Read the model definition and answer for the solid it produces. Units are mm, in the model's axes. A direction names the side the tool comes from. Coordinates: 2 decimals unless noted, no trailing zeros. Loops run counter-clockwise (first coordinate to the right, second up) from the corner with the lowest first, then second, coordinate; pieces in that order, holes last. Notation, with made-up numbers: (74.5, 32) - (116.5, 32) arc R17 ccw to (116.5, 39) - close; hole circle Ø2 at (-36, 74.5). An arc over 180 degrees is marked (long way). Use one line per item in the form item = value.
from build123d import *

# Parameters (mm, degrees)
SKETCH1_W            = 81.28
SKETCH1_H            = 81.28
SKETCH1_W_2          = 76.2
SKETCH1_H_2          = 76.2
BOSS_EXTRUDE1_DEPTH  = 177.8
SKETCH2_W            = 2.54
SKETCH2_H            = 38.1
BOSS_EXTRUDE2_DEPTH  = 25.4
SKETCH3_W            = 2.54
SKETCH3_H            = 25.4
CUT_EXTRUDE1_DEPTH   = 212.720846399
BOSS_EXTRUDE3_DEPTH  = 12.7
BOSS_EXTRUDE4_DEPTH  = 12.7
SKETCH14_W           = 5.08
SKETCH14_H           = 25.4
BOSS_EXTRUDE6_DEPTH  = 76.2
CUT_EXTRUDE2_REACH   = 243.407
SKETCH16_W           = 23.13
SKETCH16_H           = 20.32
SKETCH22_R           = 2
CUT_EXTRUDE6_DEPTH   = 252.036309724
SKETCH28_W           = 35.399999812
SKETCH28_H           = 50.8
BOSS_EXTRUDE7_DEPTH  = 38.1
CUT_EXTRUDE8_REACH   = 246.574
SKETCH32_W           = 33.02
SKETCH32_H           = 30.319999812
CUT_EXTRUDE9_DEPTH   = 25.4
CUT_EXTRUDE13_REACH  = 245.27
SKETCH34_R           = 9.890000016
BOSS_EXTRUDE9_DEPTH  = 2.54
SKETCH38_W           = 2.54
SKETCH38_H           = 25.4
CUT_EXTRUDE15_DEPTH  = 63.5
CUT_EXTRUDE17_REACH  = 224.71
SKETCH40_R           = 2.999995
SKETCH41_R           = 3.77
SKETCH41_R_2         = 2.5
BOSS_EXTRUDE10_DEPTH = 5
BOSS_EXTRUDE11_START = 5
SKETCH42_R           = 3.77
SKETCH42_R_2         = 2.5
BOSS_EXTRUDE11_DEPTH = 5
SKETCH43_W           = 76.2
SKETCH43_H           = 76.2
CUT_EXTRUDE20_DEPTH  = 25.4
SKETCH44_W           = 174.6
SKETCH44_H           = 70
SKETCH44_R           = 1.5
BOSS_EXTRUDE12_DEPTH = 2.54
FILLET1_R            = 5.08
FILLET2_R            = 12.7
FILLET3_R            = 2.54
FILLET7_R            = 12.7
FILLET9_R            = 12.7
BOSS_EXTRUDE20_DEPTH = 88.9
CUT_EXTRUDE21_REACH  = 275.109
SKETCH54_R           = 2.5
SKETCH55_W           = 30.48
SKETCH55_H           = 33.02
BOSS_EXTRUDE21_DEPTH = 2.54
FILLET12_R           = 2.54
FILLET13_R           = 2.54


with BuildPart() as part:
    # Sketch1 → Boss-Extrude1 (new body)
    with BuildSketch(Plane(origin=(0, 0, 0), x_dir=(1, 0, 0), z_dir=(0, 1, 0))):
        with Locations((40.64, 40.64)):
            Rectangle(SKETCH1_W, SKETCH1_H)
        with Locations((40.64, 40.64)):
            Rectangle(SKETCH1_W_2, SKETCH1_H_2, mode=Mode.SUBTRACT)
    extrude(amount=BOSS_EXTRUDE1_DEPTH)

    # Sketch2 → Boss-Extrude2 (add)
    with BuildSketch(Plane(origin=(0, 0, 0), x_dir=(0, 0, -1), z_dir=(1, 0, 0))):
        with Locations((64.77, 19.05)):
            Rectangle(SKETCH2_W, SKETCH2_H)
    extrude(amount=-BOSS_EXTRUDE2_DEPTH)

    # Sketch3 → Cut-Extrude1 (cut, through all)
    with BuildSketch(Plane.XY):
        with Locations((80.01, 12.7)):
            Rectangle(SKETCH3_W, SKETCH3_H)
    extrude(amount=-CUT_EXTRUDE1_DEPTH, mode=Mode.SUBTRACT)

    # Sketch7 → Boss-Extrude3 (add)
    with BuildSketch(Plane.XY):
        Polygon((81.28, 25.4), (106.68, 50.8), (81.28, 50.8), align=None)
    extrude(amount=-BOSS_EXTRUDE3_DEPTH)

    # Sketch10 → Boss-Extrude4 (add)
    with BuildSketch(Plane(origin=(0, 0, -81.28), x_dir=(-1, 0, 0), z_dir=(0, 0, -1))):
        Polygon((-81.28, 25.4), (-81.28, 50.8), (-106.68, 50.8), align=None)
    extrude(amount=-BOSS_EXTRUDE4_DEPTH)

    # Sketch14 → Boss-Extrude6 (add)
    with BuildSketch(Plane(origin=(81.28, 0, 0), x_dir=(0, 0, -1), z_dir=(1, 0, 0))):
        with Locations((40.64, 38.1)):
            Rectangle(SKETCH14_W, SKETCH14_H)
    extrude(amount=BOSS_EXTRUDE6_DEPTH)

    # Sketch16 → Cut-Extrude2 (cut, up to next)
    with BuildSketch(Plane.XY.offset(-38.1), mode=Mode.PRIVATE) as cut_extrude2_sk1:
        with Locations((129.405, 40.64)):
            Rectangle(SKETCH16_W, SKETCH16_H)
    cut_extrude2_tool1 = extrude(cut_extrude2_sk1.sketch, amount=-CUT_EXTRUDE2_REACH, mode=Mode.PRIVATE) & part.part
    add(cut_extrude2_tool1.solids().sort_by_distance((129.405, 40.64, -38.1))[0], mode=Mode.SUBTRACT)

    # Sketch22 → Cut-Extrude6 (cut, through all)
    with BuildSketch(Plane.XY):
        with Locations((93.98, 45.72)):
            Circle(SKETCH22_R)
    extrude(amount=-CUT_EXTRUDE6_DEPTH, mode=Mode.SUBTRACT)

    # Sketch28 → Boss-Extrude7 (add)
    with BuildSketch(Plane(origin=(81.28, 0, 0), x_dir=(0, 0, -1), z_dir=(1, 0, 0))):
        with Locations((40.64, 152.4)):
            Rectangle(SKETCH28_W, SKETCH28_H)
    extrude(amount=BOSS_EXTRUDE7_DEPTH)

    # Sketch30 → Cut-Extrude8 (cut, up to next)
    with BuildSketch(Plane.XY.offset(-22.940000094), mode=Mode.PRIVATE) as cut_extrude8_sk1:
        Polygon((81.28, 127), (119.38, 127), (119.38, 152.4), align=None)
    cut_extrude8_tool1 = extrude(cut_extrude8_sk1.sketch, amount=-CUT_EXTRUDE8_REACH, mode=Mode.PRIVATE) & part.part
    add(cut_extrude8_tool1.solids().sort_by_distance((106.68, 135.466667, -22.94))[0], mode=Mode.SUBTRACT)

    # Sketch32 → Cut-Extrude9 (cut)
    with BuildSketch(Plane(origin=(0, 177.8, 0), x_dir=(1, 0, 0), z_dir=(0, 1, 0))):
        with Locations((100.33, 40.64)):
            Rectangle(SKETCH32_W, SKETCH32_H)
    extrude(amount=-CUT_EXTRUDE9_DEPTH, mode=Mode.SUBTRACT)

    # Cut-Extrude13: up to this face of the body (flat: up to its plane)
    cut_extrude13_end = Plane(part.part.faces().sort_by_distance((78.74, 101.6, -40.64))[0])
    # Sketch34 → Cut-Extrude13 (cut, up to the picked face)
    with BuildSketch(Plane(origin=(119.38, 0, 0), x_dir=(0, 0, -1), z_dir=(1, 0, 0)), mode=Mode.PRIVATE) as cut_extrude13_sk1:
        with Locations(Location((40.593000094, 165.1, 0), (0, 0, 180))):
            Circle(SKETCH34_R)
    cut_extrude13_tool1 = split(extrude(cut_extrude13_sk1.sketch, amount=-CUT_EXTRUDE13_REACH, mode=Mode.PRIVATE), bisect_by=cut_extrude13_end, keep=Keep.BOTH, mode=Mode.PRIVATE)
    add(cut_extrude13_tool1.solids().sort_by(Axis((119.38, 165.1, -40.593), (-1, 0, 0)))[0], mode=Mode.SUBTRACT)

    # Sketch37 → Boss-Extrude9 (add)
    with BuildSketch(Plane.XY.offset(-63.5)):
        Polygon((-25.4, 38.1), (0, 38.1), (0, 52.764696837), align=None)
    extrude(amount=-BOSS_EXTRUDE9_DEPTH)

    # Sketch38 → Cut-Extrude15 (cut)
    with BuildSketch(Plane.XY):
        with Locations((1.27, 12.7)):
            Rectangle(SKETCH38_W, SKETCH38_H)
    extrude(amount=-CUT_EXTRUDE15_DEPTH, mode=Mode.SUBTRACT)

    # Cut-Extrude17: up to this face of the body (flat: up to its plane)
    cut_extrude17_end = Plane(part.part.faces().sort_by_distance((0, 99.23335202, -41.514066738))[0])
    # Sketch40 → Cut-Extrude17 (cut, up to the picked face)
    with BuildSketch(Plane(origin=(81.28, 0, 0), x_dir=(0, 0, -1), z_dir=(1, 0, 0)), mode=Mode.PRIVATE) as cut_extrude17_sk1:
        with Locations((19.05, 101.6)):
            Circle(SKETCH40_R)
    cut_extrude17_tool1 = split(extrude(cut_extrude17_sk1.sketch, amount=-CUT_EXTRUDE17_REACH, mode=Mode.PRIVATE), bisect_by=cut_extrude17_end, keep=Keep.BOTH, mode=Mode.PRIVATE)
    # Sketch40 → Cut-Extrude17 (cut, up to the picked face)
    with BuildSketch(Plane(origin=(81.28, 0, 0), x_dir=(0, 0, -1), z_dir=(1, 0, 0)), mode=Mode.PRIVATE) as cut_extrude17_sk2:
        with Locations((62.23, 101.6)):
            Circle(SKETCH40_R)
    cut_extrude17_tool2 = split(extrude(cut_extrude17_sk2.sketch, amount=-CUT_EXTRUDE17_REACH, mode=Mode.PRIVATE), bisect_by=cut_extrude17_end, keep=Keep.BOTH, mode=Mode.PRIVATE)
    add(cut_extrude17_tool1.solids().sort_by(Axis((81.28, 101.6, -19.05), (-1, 0, 0)))[0], mode=Mode.SUBTRACT)
    add(cut_extrude17_tool2.solids().sort_by(Axis((81.28, 101.6, -62.23), (-1, 0, 0)))[0], mode=Mode.SUBTRACT)

    # Sketch41 → Boss-Extrude10 (add)
    # profile 1 of 2: a face of its own
    with BuildSketch(Plane(origin=(81.28, 0, 0), x_dir=(0, 0, -1), z_dir=(1, 0, 0))):
        with Locations(Location((19.05, 101.6, 0), (0, 0, 180))):
            Circle(SKETCH41_R)
        with Locations((19.05, 101.6)):
            Circle(SKETCH41_R_2, mode=Mode.SUBTRACT)
    # profile 2 of 2: a face of its own
    with BuildSketch(Plane(origin=(81.28, 0, 0), x_dir=(0, 0, -1), z_dir=(1, 0, 0))):
        with Locations(Location((62.23, 101.6, 0), (0, 0, 180))):
            Circle(SKETCH41_R)
        with Locations((62.23, 101.6)):
            Circle(SKETCH41_R_2, mode=Mode.SUBTRACT)
    extrude(amount=BOSS_EXTRUDE10_DEPTH)

    # Sketch42 → Boss-Extrude11 (add)
    # profile 1 of 2: a face of its own
    with BuildSketch(Plane.ZY.offset(BOSS_EXTRUDE11_START)):
        with Locations((-62.23, 101.6)):
            Circle(SKETCH42_R)
        with Locations(Location((-62.23, 101.6, 0), (0, 0, 180))):
            Circle(SKETCH42_R_2, mode=Mode.SUBTRACT)
    # profile 2 of 2: a face of its own
    with BuildSketch(Plane.ZY.offset(BOSS_EXTRUDE11_START)):
        with Locations((-19.05, 101.6)):
            Circle(SKETCH42_R)
        with Locations(Location((-19.05, 101.6, 0), (0, 0, 180))):
            Circle(SKETCH42_R_2, mode=Mode.SUBTRACT)
    extrude(amount=-BOSS_EXTRUDE11_DEPTH)

    # Sketch43 → Cut-Extrude20 (cut)
    with BuildSketch(Plane(origin=(0, 177.8, 0), x_dir=(1, 0, 0), z_dir=(0, 1, 0))):
        Polygon((83.82, 58.339999906), (83.82, 22.940000094), (81.28, 22.940000094), (81.28, 0), (0, 0), (0, 81.28), (81.28, 81.28), (81.28, 58.339999906), align=None)
        with Locations((40.64, 40.64)):
            Rectangle(SKETCH43_W, SKETCH43_H, mode=Mode.SUBTRACT)
    extrude(amount=-CUT_EXTRUDE20_DEPTH, mode=Mode.SUBTRACT)

    # Sketch44 → Boss-Extrude12 (add)
    with BuildSketch(Plane.XY):
        with Locations((87.3, 85.8)):
            Rectangle(SKETCH44_W, SKETCH44_H)
        with Locations((140.97, 115.8)):
            Circle(SKETCH44_R, mode=Mode.SUBTRACT)
        with Locations((140.97, 55.8)):
            Circle(SKETCH44_R, mode=Mode.SUBTRACT)
    extrude(amount=-BOSS_EXTRUDE12_DEPTH)

    # Fillet1
    fillet1_edges = [part.edges().sort_by_distance(p)[0] for p in [
        (106.68, 50.8, -7.62),
        (106.68, 50.8, -74.93),
    ]]
    fillet(fillet1_edges, radius=FILLET1_R)

    # Fillet2
    fillet2_edges = [part.edges().sort_by_distance(p)[0] for p in [
        (174.6, 120.8, -1.27),
        (174.6, 50.8, -1.27),
    ]]
    fillet(fillet2_edges, radius=FILLET2_R)

    # Fillet3
    fillet3_edges = [part.edges().sort_by_distance(p)[0] for p in [
        (157.48, 50.8, -40.64),
        (157.48, 25.4, -40.64),
    ]]
    fillet(fillet3_edges, radius=FILLET3_R)

    # Fillet7
    fillet7_edges = [part.edges().sort_by_distance(p)[0] for p in [
        (-25.4, 38.1, -64.77),
    ]]
    fillet(fillet7_edges, radius=FILLET7_R)

    # Fillet9
    fillet9_edges = [part.edges().sort_by_distance(p)[0] for p in [
        (83.82, 177.8, -24.210000094),
        (83.82, 177.8, -57.069999906),
    ]]
    fillet(fillet9_edges, radius=FILLET9_R)

    # Sketch53 → Boss-Extrude20 (add)
    with BuildSketch(Plane(origin=(0, 0, 0), x_dir=(-1, 0, 0), z_dir=(0, -1, 0))):
        Polygon((-35.659105782, 81.28), (-35.659105782, 78.74), (-45.72, 78.74), (-45.72, 111.76), (-15.24, 111.76), (-15.24, 106.68), (-40.64, 106.68), (-40.64, 81.28), align=None)
    extrude(amount=-BOSS_EXTRUDE20_DEPTH)

    # Sketch54 → Cut-Extrude21 (cut, up to next)
    with BuildSketch(Plane(origin=(0, 0, -111.76), x_dir=(-1, 0, 0), z_dir=(0, 0, -1)), mode=Mode.PRIVATE) as cut_extrude21_sk1:
        with Locations((-30.48, 76.2)):
            Circle(SKETCH54_R)
    cut_extrude21_tool1 = extrude(cut_extrude21_sk1.sketch, amount=-CUT_EXTRUDE21_REACH, mode=Mode.PRIVATE) & part.part
    # Sketch54 → Cut-Extrude21 (cut, up to next)
    with BuildSketch(Plane(origin=(0, 0, -111.76), x_dir=(-1, 0, 0), z_dir=(0, 0, -1)), mode=Mode.PRIVATE) as cut_extrude21_sk2:
        with Locations((-30.48, 44.45)):
            Circle(SKETCH54_R)
    cut_extrude21_tool2 = extrude(cut_extrude21_sk2.sketch, amount=-CUT_EXTRUDE21_REACH, mode=Mode.PRIVATE) & part.part
    # Sketch54 → Cut-Extrude21 (cut, up to next)
    with BuildSketch(Plane(origin=(0, 0, -111.76), x_dir=(-1, 0, 0), z_dir=(0, 0, -1)), mode=Mode.PRIVATE) as cut_extrude21_sk3:
        with Locations((-30.48, 12.7)):
            Circle(SKETCH54_R)
    cut_extrude21_tool3 = extrude(cut_extrude21_sk3.sketch, amount=-CUT_EXTRUDE21_REACH, mode=Mode.PRIVATE) & part.part
    add(cut_extrude21_tool1.solids().sort_by_distance((30.48, 76.2, -111.76))[0], mode=Mode.SUBTRACT)
    add(cut_extrude21_tool2.solids().sort_by_distance((30.48, 44.45, -111.76))[0], mode=Mode.SUBTRACT)
    add(cut_extrude21_tool3.solids().sort_by_distance((30.48, 12.7, -111.76))[0], mode=Mode.SUBTRACT)

    # Sketch55 → Boss-Extrude21 (add)
    with BuildSketch(Plane(origin=(0, 0, 0), x_dir=(-1, 0, 0), z_dir=(0, -1, 0))):
        with Locations((-30.48, 95.25)):
            Rectangle(SKETCH55_W, SKETCH55_H)
    extrude(amount=-BOSS_EXTRUDE21_DEPTH)

    # Fillet12
    fillet12_edges = [part.edges().sort_by_distance(p)[0] for p in [
        (81.28, 136.6, 0),
        (81.28, 101.6, -81.28),
        (0, 76.2, -81.28),
        (0, 88.9, 0),
    ]]
    fillet(fillet12_edges, radius=FILLET12_R)

    # Fillet13
    fillet13_edges = [part.edges().sort_by_distance(p)[0] for p in [
        (15.24, 45.72, -106.68),
        (15.24, 44.45, -111.76),
    ]]
    fillet(fillet13_edges, radius=FILLET13_R - 0.0001)  # a hair under: the kernel refuses the full size


solid = part.part
Item 1: For a pull along Y with two mould halves and no side action, classify faces 1 (the cylindrical face through (118.128, 174.755, -42.737)), 2 (the cylindrical face through (1.29, 102.5, -65.09)), 3 (the flat face through (86.28, 102, -22)), 4 (the cylindrical face through (170.78, 54.42, -1.29)) as +Y half, -Y half, draft (parallel to the pull), parting line (faces both ways), or undercut.
Results below:
face_1 = undercut
face_2 = undercut
face_3 = draft
face_4 = -Y half
Item 2: Which of the six approach directions +Z, -Z, +X, -X, +Y, -Y give full straight-line access (tool end or side, diameter ignored) to faces 5 (the flat face through (52, 75, -81.28)), 6 (the cylindrical face through (-2.54, 105.34, -19.54)), 7 (the flat face through (36, 88.9, -108)), 8 (the flat face through (100, 165, -25.48)), 9 (the cylindrical face through (99.14, 47.59, -7.69))?
Results below:
face_5 = +Y
face_6 = -X
face_7 = -Z, +X, -X, +Y
face_8 = -X, +Y
face_9 = +X
Item 3: The part is cut by section A-A on x = 12.5. Give the vertices of the cut face in (y, z), plus the area to 3 significant figures.
Results below:
outline = (0, -81.28) - (152.4, -81.28) - (152.4, -78.74) - (0, -78.74) - close; (0, -2.54) - (152.4, -2.54) - (152.4, 0) - (0, 0) - close
area = 774 mm²
Item 4: The part is cut by section C-C on z = -47. Give the vertices of the cut face in (x, y).
Results below:
outline = (0, 25.4) - (2.54, 25.4) - (2.54, 152.4) - (0, 152.4) - close; (78.74, 25.4) - (81.28, 25.4) - (81.28, 127) - (119.38, 152.4) - (119.38, 157.57) - (116.84, 157.57) - (116.84, 152.4) - (78.74, 152.4) - close; (116.84, 172.63) - (119.38, 172.63) - (119.38, 177.8) - (116.84, 177.8) - close
Item 5: Each of these flat-tipped pins is pushed along its axis until it touches: P1, Ø2.5, axis at y = 103.5, z = -62.5, coming from the +X side; P2, Ø1, axis at y = 32.5, z = -31, coming from the -X side; P3, Ø10, axis at x = 55.5, y = 71.5, coming from the -Z side; P4, Ø2.5, axis at x = 140.97, y = 115.8, coming from the +Z side. Where does it stop, or does it pass through?
Results below:
P1 = 86.28
P2 = 0
P3 = -81.28
P4 = through
Item 6: Find the intervals of material crossed by L1, parallel to X at y = 64, z = -38; L2, parallel to Z at x = 10, y = 79; L3, parallel to Z at x = 40.5, y = 25.5, in increasing order.
Results below:
L1 = 0 to 2.54, 78.74 to 81.28
L2 = -81.28 to -78.74, -2.54 to 0
L3 = -111.76 to -106.68, -81.28 to -78.74, -2.54 to 0
Item 7: The part is cut by section B-B on y = 76.2. Count the separate pieces of the cut face and the enclosed holes in it, plus the area to 3 significant figures.
Results below:
separate_pieces = 2
enclosed_holes = 1
area = 1,290 mm²
